Could you check a few things on this model? Use its own coordinates, in mm. A direction names the side the tool comes from. Coordinates: 2 decimals unless noted, no trailing zeros. Order: outer loops, then holes, each group sorted by start corner. A loop starts at its lowest first (then second) coordinate and runs counter-clockwise, first axis right, second up. Notation, with made-up numbers: (-34.5, -30.5) -> (-6.5, -30.5) arc R16 cw to (-6.5, -15.5) -> close; hole circle Ø8 at (49.25, 38.25). An arc over 180 degrees is marked (long way). Use a Markdown table: item, result. Add a question column.
1) Thinking about a two-plate mould opening in X: for faces 3 (the cylindrical face through (-22.513, 2.028, -5.195)), 4 (the flat face through (45.75, 2, 0)), 5 (the flat face through (-1, 2, -15)), 6 (the flat face through (-45.75, 2, 0)), which applies, +X half, -X half, draft (parallel to the pull), parting line (faces both ways), or undercut?
2) If I drill on L1, parallel to X at y = 0.95, z = 0; L2, parallel to Z at x = 4.5, y = 2.55; L3, parallel to X at y = 1.9, z = 5, over which ranges is the centre line in solid material (lowest first)? Write a range as [from, to].
3) If we section it at A-A (x = 6): Write out the boundary of the cut face in (y, z).
4) If we section it at B-B (z = 5): Write out the boundary of the cut face in (x, y).
5) Which directions (+Z, -Z, +X, -X, +Y, -Y) give clear straight access to the entire face, cutting with the end or side of a thin tool? Please do faces 1 (the flat face through (-1, 2, 15)), 2 (the flat face through (-21, 2, 0)).
6) If we section it at D-D (y = 1.1): Write out the boundary of the cut face in (x, z), plus the area to 3 significant figures.
7) If we section it at C-C (x = 24): Write out the boundary of the cut face in (y, z), plus the area to 3 significant figures.
```python
from build123d import *

# Parameters (mm, degrees)
SKETCH1_W           = 91.5
SKETCH1_H           = 30
SKETCH1_R           = 2
SKETCH1_W_2         = 42
SKETCH1_H_2         = 20
BOSS_EXTRUDE1_DEPTH = 4
SKETCH2_R           = 1.5
CUT_EXTRUDE1_DEPTH  = 49.312136156


with BuildPart() as part:
    # Sketch1 → Boss-Extrude1 (new body)
    with BuildSketch(Plane(origin=(0, 0, 0), x_dir=(1, 0, 0), z_dir=(0, 1, 0))):
        Rectangle(SKETCH1_W, SKETCH1_H)
        with Locations(Location((-39.75, 0, 0), (0, 0, 270))):
            Circle(SKETCH1_R, mode=Mode.SUBTRACT)
        with Locations(Location((39.75, 0, 0), (0, 0, 90))):
            Circle(SKETCH1_R, mode=Mode.SUBTRACT)
        Rectangle(SKETCH1_W_2, SKETCH1_H_2, mode=Mode.SUBTRACT)
    extrude(amount=BOSS_EXTRUDE1_DEPTH)

    # Sketch2 → Cut-Extrude1 (cut, through all)
    with BuildSketch(Plane(origin=(0, 4, 0), x_dir=(1, 0, 0), z_dir=(0, 1, 0))):
        with Locations(Location((-24, 5, 0), (0, 0, 270))):
            Circle(SKETCH2_R)
        with Locations(Location((-24, -5, 0), (0, 0, 90))):
            Circle(SKETCH2_R)
        with Locations(Location((24, -5, 0), (0, 0, 270))):
            Circle(SKETCH2_R)
        with Locations(Location((24, 5, 0), (0, 0, 90))):
            Circle(SKETCH2_R)
    extrude(amount=-CUT_EXTRUDE1_DEPTH, mode=Mode.SUBTRACT)


solid = part.part
```
Answer sheet:
| question | item | result |
|---|---|---|
| 1 | face 3 | undercut |
| 1 | face 4 | +X half |
| 1 | face 5 | draft |
| 1 | face 6 | -X half |
| 2 | L1 | [-45.75, -41.75], [-37.75, -21], [21, 37.75], [41.75, 45.75] |
| 2 | L2 | [-15, -10], [10, 15] |
| 2 | L3 | [-45.75, -25.5], [-22.5, -21], [21, 22.5], [25.5, 45.75] |
| 3 | outline | (0, -15) -> (4, -15) -> (4, -10) -> (0, -10) -> close; (0, 10) -> (4, 10) -> (4, 15) -> (0, 15) -> close |
| 4 | outline | (-45.75, 0) -> (-25.5, 0) -> (-25.5, 4) -> (-45.75, 4) -> close; (-22.5, 0) -> (-21, 0) -> (-21, 4) -> (-22.5, 4) -> close; (21, 0) -> (22.5, 0) -> (22.5, 4) -> (21, 4) -> close; (25.5, 0) -> (45.75, 0) -> (45.75, 4) -> (25.5, 4) -> close |
| 5 | face 1 | +Z, +X, -X, +Y, -Y |
| 5 | face 2 | +Y, -Y |
| 6 | outline | (-45.75, -15) -> (45.75, -15) -> (45.75, 15) -> (-45.75, 15) -> close; hole circle Ø4 at (-39.75, 0); hole circle Ø3 at (-24, -5); hole circle Ø3 at (-24, 5); hole (-21, -10) -> (21, -10) -> (21, 10) -> (-21, 10) -> close; hole circle Ø3 at (24, -5); hole circle Ø3 at (24, 5); hole circle Ø4 at (39.75, 0) |
| 6 | area | 1,850 mm2 |
| 7 | outline | (0, -15) -> (4, -15) -> (4, -6.5) -> (0, -6.5) -> close; (0, -3.5) -> (4, -3.5) -> (4, 3.5) -> (0, 3.5) -> close; (0, 6.5) -> (4, 6.5) -> (4, 15) -> (0, 15) -> close |
| 7 | area | 96.0 mm2 |
